from build123d import *

# Parameters (mm, degrees)
SKETCH_2_W          = 230
SKETCH_2_H          = 152
SKETCH_2_W_2        = 73
SKETCH_2_H_2        = 138
SKETCH_2_W_3        = 142
SKETCH_2_H_3        = 142
EXTRUDE_2_DEPTH     = 10
SKETCH_3_W          = 73
SKETCH_3_H          = 138
EXTRUDE_3_DEPTH     = 12
SKETCH_4_R          = 1.6
SKETCH_4_R_2        = 2.201608842
CUT_EXTRUDE_1_DEPTH = 140.58868149


with BuildPart() as part:
    # Sketch 2 → Extrude 2 (new body)
    # profile 1 of 3: a face of its own
    with BuildSketch(Plane(origin=(0, 0, 0), x_dir=(1, 0, 0), z_dir=(0, 1, 0))):
        Rectangle(SKETCH_2_W, SKETCH_2_H)
        with Locations((-73.5, 2)):
            Rectangle(SKETCH_2_W_2, SKETCH_2_H_2, mode=Mode.SUBTRACT)
        with Locations((39, 0)):
            Rectangle(SKETCH_2_W_3, SKETCH_2_H_3, mode=Mode.SUBTRACT)
    # profile 2 of 3: a face of its own
    with BuildSketch(Plane(origin=(0, 0, 0), x_dir=(1, 0, 0), z_dir=(0, 1, 0))):
        with Locations((39, 0)):
            Rectangle(SKETCH_2_W_3, SKETCH_2_H_3)
    # profile 3 of 3: a face of its own
    with BuildSketch(Plane(origin=(0, 0, 0), x_dir=(1, 0, 0), z_dir=(0, 1, 0))):
        with Locations((-73.5, 2)):
            Rectangle(SKETCH_2_W_2, SKETCH_2_H_2)
    extrude(amount=EXTRUDE_2_DEPTH)

    # Sketch 3 → Extrude 3 (add)
    with BuildSketch(Plane(origin=(0, 10, 0), x_dir=(1, 0, 0), z_dir=(0, 1, 0))):
        with Locations((-73.5, 2)):
            Rectangle(SKETCH_3_W, SKETCH_3_H)
    extrude(amount=EXTRUDE_3_DEPTH)

    # Sketch 4 → Cut-Extrude 1 (cut, through all)
    with BuildSketch(Plane.XZ):
        with Locations(Location((0, 73.5, 0), (0, 0, 270))):
            Circle(SKETCH_4_R)
        with Locations(Location((112.5, -55, 0), (0, 0, 270))):
            Circle(SKETCH_4_R)
        with Locations(Location((112.5, 71, 0), (0, 0, 270))):
            Circle(SKETCH_4_R)
        with Locations(Location((-112.5, -51, 0), (0, 0, 270))):
            Circle(SKETCH_4_R)
        with Locations(Location((-112.5, 71, 0), (0, 0, 270))):
            Circle(SKETCH_4_R_2)
    extrude(amount=-CUT_EXTRUDE_1_DEPTH, mode=Mode.SUBTRACT)


solid = part.part
Input: part model. Units: mm. Frame: model coordinates. A direction names the side the tool comes from. Give positions to 0.01 mm unless a question says otherwise; leave off trailing zeros. Write each loop counter-clockwise with the first axis right and the second up, starting at its lowest first coordinate (ties: lowest second). Pieces come first, ordered by that corner, then holes. Notation, with made-up numbers: (49, 26.5) -> (94, 26.5) arc R18 cw to (94, 53.5) -> close; hole circle Ø3 at (49, 86.25). An arc over 180 degrees is marked (long way). Use one line per item in the form item = value. Start each with the question number.
1) Pin query (flat end, axial travel): pin 1 (1.9 mm diameter, centred on x = -112.5, z = -51, fed in from -Y); pin 2 (4 mm diameter, centred on x = 0, z = 73.5, fed in from +Y); pin 3 (6 mm diameter, centred on y = 17.5, z = -32.5, fed in from -X); pin 4 (3.5 mm diameter, centred on x = -80.5, y = 18, fed in from -Z). Return the tip coordinate at first contact, or that it passes through.
2) Section query B-B on x = -69.5. Return the cut outline in (y, z), then the cut area to 3 significant figures.
3) Draft query along X for faces 1 (the flat face through (-2, 5, 76)), 2 (the flat face through (-110, 16, -1)), 3 (the cylindrical face through (-110.64, 4.93, 69.82)), 4 (the flat face through (-37, 16, -1)). Return one class per face: pulls with the +X half, pulls with the -X half, needs draft (parallel to the pull), parting line crosses it, or undercut.
4) Set-up query: faces 5 (the flat face through (-2, 0, -1)), 6 (the flat face through (-74, 16, 67)), 7 (the flat face through (-74, 16, -71)). Return all of +Z, -Z, +X, -X, +Y, -Y with unobstructed straight access to the full face (end or side cutting, diameter ignored); none if empty.
5) Section query A-A on z = -21. Return the cut outline in (x, y), then the cut area to 3 significant figures.
6) Section query C-C on y = 16.75. Return the cut outline in (x, z), then the cut area to 3 significant figures.
7) Section query D-D on x = 101.5. Return the cut outline in (y, z).
8) Ray query, probe 1 along X at (y, z) = (2.5, 71); probe 2 along Z at (x, y) = (112.5, 3.5); probe 3 along X at (y, z) = (7.5, -51). Return the intervals inside material, ascending. Write a range as from..to.
Outcome:
q1.pin_1 = through
q1.pin_2 = 10
q1.pin_3 = -110
q1.pin_4 = -71
q2.outline = (0, -76) -> (10, -76) -> (10, -71) -> (22, -71) -> (22, 67) -> (10, 67) -> (10, 76) -> (0, 76) -> close
q2.area = 3,180 mm^2
q3.face_1 = needs draft
q3.face_2 = pulls with the -X half
q3.face_3 = undercut
q3.face_4 = pulls with the +X half
q4.face_5 = +Z, -Z, +X, -X, -Y
q4.face_6 = +Z, +X, -X, +Y
q4.face_7 = -Z, +X, -X, +Y
q5.outline = (-115, 0) -> (115, 0) -> (115, 10) -> (-37, 10) -> (-37, 22) -> (-110, 22) -> (-110, 10) -> (-115, 10) -> close
q5.area = 3,180 mm^2
q6.outline = (-110, -71) -> (-37, -71) -> (-37, 67) -> (-110, 67) -> close
q6.area = 10,100 mm^2
q7.outline = (0, -76) -> (10, -76) -> (10, 76) -> (0, 76) -> close
q8.probe_1 = -115..-114.7, -110.3..110.9, 114.1..115
q8.probe_2 = -76..-56.6, -53.4..69.4, 72.6..76
q8.probe_3 = -115..-114.1, -110.9..115
